```python
from build123d import *

# Parameters (mm, degrees)
SKETCH1_R           = 2
BOSS_EXTRUDE1_DEPTH = 65
SKETCH8_R           = 2
REVOLVE4_ANGLE      = 120
BOSS_EXTRUDE3_DEPTH = 2


with BuildPart() as part:
    # Sketch1 → Boss-Extrude1 (new body)
    with BuildSketch(Plane.XY):
        Circle(SKETCH1_R)
    extrude(amount=BOSS_EXTRUDE1_DEPTH)

    # Sketch8 → Revolve4 (revolve)
    with BuildSketch(Plane(origin=(0, 0, 0), x_dir=(-1, 0, 0), z_dir=(0, 0, -1))):
        with Locations(Location((0, 0, 0), (0, 0, 90))):
            Circle(SKETCH8_R)
    revolve(axis=Axis((0, -2.964026972, 0), (-1, 0, 0)), revolution_arc=REVOLVE4_ANGLE)

    # Sketch12 → Boss-Extrude3 (add)
    with BuildSketch(Plane(origin=(0, -2.223020229, 1.283461328), x_dir=(1, 0, 0), z_dir=(0, -0.8660254037844362, 0.5000000000000042))):
        with BuildLine():
            Line((2, -4.946040459), (1.936491673, -4.946040459))
            ThreePointArc((1.936491673, -4.946040459), (0, -6.446040459), (-1.936491673, -4.946040459))
            Line((-1.936491673, -4.946040459), (-2, -4.946040459))
            Line((-2, -4.946040459), (-3, -4.946040459))
            Line((-3, -4.946040459), (-3, -3.946040459))
            Line((-3, -3.946040459), (-2, -3.946040459))
            Line((-2, -3.946040459), (-1.936491673, -3.946040459))
            ThreePointArc((-1.936491673, -3.946040459), (0, -2.446040459), (1.936491673, -3.946040459))
            Line((1.936491673, -3.946040459), (2, -3.946040459))
            Line((2, -3.946040459), (3, -3.946040459))
            Line((3, -3.946040459), (3, -4.946040459))
            Line((3, -4.946040459), (2, -4.946040459))
        make_face()
    extrude(amount=BOSS_EXTRUDE3_DEPTH)


solid = part.part
```
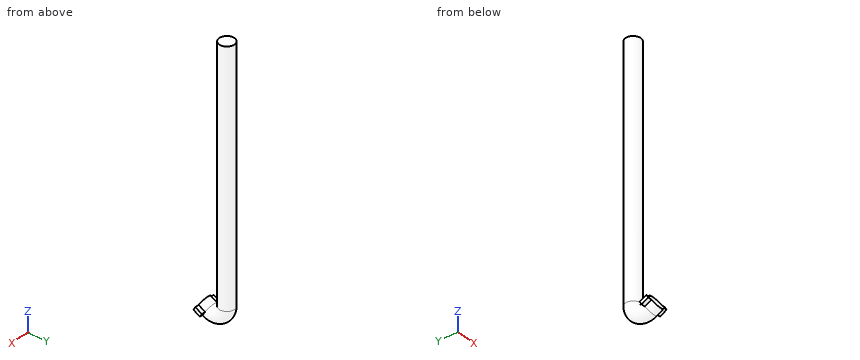
Could you check a few things on this model? Use its own coordinates, in mm. Round coordinates to 2 decimals unless told otherwise and drop trailing zeros. Loops run counter-clockwise (first coordinate to the right, second up) from the corner with the lowest first, then second, coordinate; pieces in that order, holes last. Notation, with made-up numbers: M -3.75,-22.75 L 44.25,-22.75 A33 cw 44.25,15.25 Z; hole C 25.5,-1.5 d7. An arc over 180 degrees is marked long. Answer as CSV lines item,"result".
1) For pin 1 Ø1 at (x, z) = (1, 52) entering from -Y; pin 2 Ø1.5 at (x, y) = (-2, -1.5) entering from +Z; pin 3 Ø1.5 at (x, z) = (-2.5, 45.5) entering from -Y; pin 4 Ø1.5 at (x, z) = (0.5, 12) entering from -Y, each with a flat end and sliding along its axis, tell me the tip position at first contact or that it passes through.
From the geometry:
pin 1,"y = -1.94"
pin 2,"z = 65"
pin 3,"y = -0.97"
pin 4,"y = -2"
2) Imagine slicing it at B-B on z = 49.5. List the corners of the cut face in (x, y) for me.
From the geometry:
outline,"C 0,0 d4"
3) If I drill on probe 1 along Y at (x, z) = (0.1, 32); probe 2 along Z at (x, y) = (-0.4, -4.75); probe 3 along Y at (x, z) = (1.35, 61), over which ranges is the centre line in solid material (lowest first)?
From the geometry:
probe 1,"-2 to 2"
probe 2,"-4.59 to -0.13"
probe 3,"-1.48 to 1.48"
4) Imagine slicing it at A-A on x = 1.3. List the corners of the cut face in (y, z) for me, and give its area (3 significant figures).
From the geometry:
outline,"M -6.94,-2.88 L -5.21,-3.88 A4.48 ccw 1.52,0 L 1.52,65 L -1.52,65 L -1.52,0 A1.44 cw -3.69,-1.25 L -5.42,-0.25 Z"
area,"223 mm^2"
